Geometry: final body of the model. Coordinates: model frame, mm. A direction names the side the tool comes from. Give positions to 0.01 mm unless a question says otherwise; leave off trailing zeros. Order: outer loops, then holes, each group sorted by start corner. A loop starts at its lowest first (then second) coordinate and runs counter-clockwise, first axis right, second up. Notation, with made-up numbers: (-29.75, 37) -> (-1.75, 37) arc R19 ccw to (-1.75, 60) -> close; hole circle Ø9 at (61, 45.5). An arc over 180 degrees is marked (long way). Write item = value, one per line.
```python
from build123d import *

# Parameters (mm, degrees)
SKETCH2_R           = 7.5
SKETCH2_R_2         = 2.75
BOSS_EXTRUDE1_DEPTH = 3
SKETCH3_R           = 5.6
BOSS_EXTRUDE2_DEPTH = 4
BOSS_EXTRUDE3_DEPTH = 80
SKETCH5_W           = 29.85
SKETCH5_H           = 6.5
SKETCH5_W_2         = 3.85
BOSS_EXTRUDE4_DEPTH = 80
SKETCH6_W           = 29.85
SKETCH6_H           = 6.5
SKETCH6_W_2         = 3.85
CUT_EXTRUDE1_DEPTH  = 54.2
BOSS_EXTRUDE5_DEPTH = 22.8
SKETCH8_W           = 10.25
SKETCH8_H           = 10
SKETCH8_R           = 2.75
BOSS_EXTRUDE6_DEPTH = 5
BOSS_EXTRUDE7_DEPTH = 5
FILLET1_R           = 2.5


with BuildPart() as part:
    # Sketch2 → Boss-Extrude1 (new body)
    # profile 1 of 4: a face of its own
    with BuildSketch(Plane.XY):
        with Locations((-20, -30)):
            Circle(SKETCH2_R)
        with Locations((-20, -30)):
            Circle(SKETCH2_R_2, mode=Mode.SUBTRACT)
    # profile 2 of 4: a face of its own
    with BuildSketch(Plane.XY):
        with BuildLine():
            Line((12.5, -22.5), (-20, -22.5))
            ThreePointArc((-20, -22.5), (-14.696699141, -24.696699141), (-12.5, -30))
            ThreePointArc((-12.5, -30), (-14.696699141, -35.303300859), (-20, -37.5))
            Line((-20, -37.5), (20, -37.5))
            ThreePointArc((20, -37.5), (14.696699141, -35.303300859), (12.5, -30))
            Line((12.5, -30), (12.5, -22.5))
        make_face()
    # profile 3 of 4: a face of its own
    with BuildSketch(Plane.XY):
        with Locations((20, -30)):
            Circle(SKETCH2_R)
        with Locations((20, -30)):
            Circle(SKETCH2_R_2, mode=Mode.SUBTRACT)
    # profile 4 of 4: a face of its own
    with BuildSketch(Plane.XY):
        with BuildLine():
            Line((20, -22.5), (12.5, -22.5))
            Line((12.5, -22.5), (12.5, -30))
            ThreePointArc((12.5, -30), (14.696699141, -24.696699141), (20, -22.5))
        make_face()
    extrude(amount=BOSS_EXTRUDE1_DEPTH)

    # Sketch3 → Boss-Extrude2 (add)
    # profile 1 of 14: a face of its own
    with BuildSketch(Plane.XY.offset(3)):
        with BuildLine():
            Line((-14.4, -26.766838493), (-17.199999967, -25.150257758))
            ThreePointArc((-17.199999967, -25.150257758), (-15.150257729, -27.200000016), (-14.4, -30))
            Line((-14.4, -30), (-14.4, -26.766838493))
        make_face()
    # profile 2 of 14: a face of its own
    with BuildSketch(Plane.XY.offset(3)):
        with Locations((-20, -30)):
            Circle(SKETCH3_R)
        Polygon((-15.9, -27.632863896), (-20, -25.265727793), (-24.1, -27.632863896), (-24.1, -32.367136104), (-20, -34.734272207), (-15.9, -32.367136104), align=None, mode=Mode.SUBTRACT)
    # profile 3 of 14: a face of its own
    with BuildSketch(Plane.XY.offset(3)):
        with BuildLine():
            Line((-17.199999967, -25.150257758), (-20, -23.533676985))
            Line((-20, -23.533676985), (-22.800000033, -25.150257758))
            ThreePointArc((-22.800000033, -25.150257758), (-20, -24.4), (-17.199999967, -25.150257758))
        make_face()
    # profile 4 of 14: a face of its own
    with BuildSketch(Plane.XY.offset(3)):
        with BuildLine():
            ThreePointArc((-25.6, -30), (-24.849742271, -27.200000016), (-22.800000033, -25.150257758))
            Line((-22.800000033, -25.150257758), (-25.6, -26.766838493))
            Line((-25.6, -26.766838493), (-25.6, -30))
        make_face()
    # profile 5 of 14: a face of its own
    with BuildSketch(Plane.XY.offset(3)):
        with BuildLine():
            ThreePointArc((-22.800000033, -34.849742242), (-24.849742271, -32.799999984), (-25.6, -30))
            Line((-25.6, -30), (-25.6, -33.233161507))
            Line((-25.6, -33.233161507), (-22.800000033, -34.849742242))
        make_face()
    # profile 6 of 14: a face of its own
    with BuildSketch(Plane.XY.offset(3)):
        with BuildLine():
            ThreePointArc((-17.199999967, -34.849742242), (-20, -35.6), (-22.800000033, -34.849742242))
            Line((-22.800000033, -34.849742242), (-20, -36.466323015))
            Line((-20, -36.466323015), (-17.199999967, -34.849742242))
        make_face()
    # profile 7 of 14: a face of its own
    with BuildSketch(Plane.XY.offset(3)):
        with BuildLine():
            Line((-14.4, -33.233161507), (-14.4, -30))
            ThreePointArc((-14.4, -30), (-15.150257729, -32.799999984), (-17.199999967, -34.849742242))
            Line((-17.199999967, -34.849742242), (-14.4, -33.233161507))
        make_face()
    # profile 8 of 14: a face of its own
    with BuildSketch(Plane.XY.offset(3)):
        with BuildLine():
            Line((25.6, -26.766838493), (22.800000033, -25.150257758))
            ThreePointArc((22.800000033, -25.150257758), (24.849742271, -27.200000016), (25.6, -30))
            Line((25.6, -30), (25.6, -26.766838493))
        make_face()
    # profile 9 of 14: a face of its own
    with BuildSketch(Plane.XY.offset(3)):
        with Locations((20, -30)):
            Circle(SKETCH3_R)
        Polygon((24.1, -27.632863896), (20, -25.265727793), (15.9, -27.632863896), (15.9, -32.367136104), (20, -34.734272207), (24.1, -32.367136104), align=None, mode=Mode.SUBTRACT)
    # profile 10 of 14: a face of its own
    with BuildSketch(Plane.XY.offset(3)):
        with BuildLine():
            Line((22.800000033, -25.150257758), (20, -23.533676985))
            Line((20, -23.533676985), (17.199999967, -25.150257758))
            ThreePointArc((17.199999967, -25.150257758), (20, -24.4), (22.800000033, -25.150257758))
        make_face()
    # profile 11 of 14: a face of its own
    with BuildSketch(Plane.XY.offset(3)):
        with BuildLine():
            ThreePointArc((14.4, -30), (15.150257729, -27.200000016), (17.199999967, -25.150257758))
            Line((17.199999967, -25.150257758), (14.4, -26.766838493))
            Line((14.4, -26.766838493), (14.4, -30))
        make_face()
    # profile 12 of 14: a face of its own
    with BuildSketch(Plane.XY.offset(3)):
        with BuildLine():
            ThreePointArc((17.199999967, -34.849742242), (15.150257729, -32.799999984), (14.4, -30))
            Line((14.4, -30), (14.4, -33.233161507))
            Line((14.4, -33.233161507), (17.199999967, -34.849742242))
        make_face()
    # profile 13 of 14: a face of its own
    with BuildSketch(Plane.XY.offset(3)):
        with BuildLine():
            ThreePointArc((22.799999796, -34.849742379), (19.999999863, -35.6), (17.199999967, -34.849742242))
            Line((17.199999967, -34.849742242), (20, -36.466323015))
            Line((20, -36.466323015), (22.799999796, -34.849742379))
        make_face()
    # profile 14 of 14: a face of its own
    with BuildSketch(Plane.XY.offset(3)):
        with BuildLine():
            Line((25.6, -33.233161507), (25.6, -30))
            ThreePointArc((25.6, -30), (24.849742202, -32.800000102), (22.799999796, -34.849742379))
            Line((22.799999796, -34.849742379), (25.6, -33.233161507))
        make_face()
    extrude(amount=BOSS_EXTRUDE2_DEPTH)

    # Sketch4 → Boss-Extrude3 (add)
    with BuildSketch(Plane.XY.offset(3)):
        Polygon((-14.4, -26.766838493), (-14.4, -22.5), (-11.4, -22.5), (-11.4, -37.5), (-14.4, -37.5), align=None)
        Polygon((14.4, -30), (14.4, -22.5), (11.4, -22.5), (11.4, -37.5), (14.4, -37.5), align=None)
    extrude(amount=BOSS_EXTRUDE3_DEPTH)

    # Sketch5 → Boss-Extrude4 (add)
    with BuildSketch(Plane.ZY.offset(-11.4)):
        with Locations((63.075, -34.25)):
            Rectangle(SKETCH5_W, SKETCH5_H)
        with Locations((42.925, -34.25)):
            Rectangle(SKETCH5_W_2, SKETCH5_H)
    extrude(amount=BOSS_EXTRUDE4_DEPTH)

    # Sketch6 → Cut-Extrude1 (cut)
    with BuildSketch(Plane.ZY.offset(68.6)):
        with Locations((63.075, -34.25)):
            Rectangle(SKETCH6_W, SKETCH6_H)
        with Locations((42.925, -34.25)):
            Rectangle(SKETCH6_W_2, SKETCH6_H)
    extrude(amount=-CUT_EXTRUDE1_DEPTH, mode=Mode.SUBTRACT)

    # Sketch7 → Boss-Extrude5 (add)
    with BuildSketch(Plane.ZY.offset(-11.4)):
        Polygon((78, -31), (78, -22.5), (83, -22.5), (83, -37.5), (78, -37.5), align=None)
    extrude(amount=BOSS_EXTRUDE5_DEPTH)

    # Sketch8 → Boss-Extrude6 (add)
    # profile 1 of 2: a face of its own
    with BuildSketch(Plane.XZ.offset(22.5)):
        with Locations((-19.525, 59.5)):
            Rectangle(SKETCH8_W, SKETCH8_H)
        with Locations((-19.525, 59.5)):
            Circle(SKETCH8_R, mode=Mode.SUBTRACT)
    # profile 2 of 2: a face of its own
    with BuildSketch(Plane.XZ.offset(22.5)):
        with Locations((19.525, 59.5)):
            Rectangle(SKETCH8_W, SKETCH8_H)
        with Locations((19.525, 59.5)):
            Circle(SKETCH8_R, mode=Mode.SUBTRACT)
    extrude(amount=BOSS_EXTRUDE6_DEPTH)

    # Sketch10 → Boss-Extrude7 (add)
    with BuildSketch(Plane(origin=(0, -22.5, 0), x_dir=(1, 0, 0), z_dir=(0, 1, 0))):
        Polygon((-10, -38.8), (10, -38.8), (11.4, -38.8), (11.4, -35.8), (-11.4, -35.8), (-11.4, -38.8), align=None)
    extrude(amount=-BOSS_EXTRUDE7_DEPTH)

    # Fillet1
    fillet1_edges = [part.edges().sort_by_distance(p)[0] for p in [
        (-14.4, -30, 83),
        (14.4, -30, 83),
    ]]
    fillet(fillet1_edges, radius=FILLET1_R)


solid = part.part
```
1) Section query D-D (z = 11.5). Output: boundary loops of the cut face in (x, y), plus the area to 3 significant figures.
Check sheet entries:
outline = (-14.4, -37.5) -> (-11.4, -37.5) -> (-11.4, -22.5) -> (-14.4, -22.5) -> close; (11.4, -37.5) -> (14.4, -37.5) -> (14.4, -22.5) -> (11.4, -22.5) -> close
area = 90.0 mm²
2) Section query A-A (y = -28.75). Count the separate pieces of the cut face and the enclosed holes in it, plus the area to 3 significant figures.
Check sheet entries:
separate_pieces = 3
enclosed_holes = 1
area = 750 mm²
3) First-contact query: P1, Ø1, axis at y = -32.5, z = 70, coming from the -X side; P2, Ø5, axis at x = 13, y = -28, coming from the -Z side; P3, Ø1, axis at y = -32, z = 12, coming from the +X side; P4, Ø3, axis at x = -0.5, z = 42.5, coming from the +Y side. Flat tips, straight axial feed; report the tip coordinate or a pass-through.
Check sheet entries:
P1 = -14.4
P2 = 0
P3 = 14.4
P4 = -31
4) Reachability of faces 4 (the face through (26, -29, 3)), 5 (the face through (0, -34, 48.15)), 6 (the face through (19, -25, 54.5)) from +Z, -Z, +X, -X, +Y, -Y: full face, straight path, thin tool, end or side. Return the list, or none.
Check sheet entries:
face_4 = none
face_5 = +Y, -Y
face_6 = +X, +Y, -Y
5) Mould query, pull axis X, two halves, no side actions, for faces 1 (the face through (-18, -26, 7)), 2 (the face through (22.02, -33.57, 4.97)), 3 (the face through (-13.687, -30.105, 82.248)). Classes: +X half, -X half, draft (parallel to the pull), parting line (faces both ways), or undercut.
Check sheet entries:
face_1 = draft
face_2 = undercut
face_3 = -X half
6) Section query B-B (x = -5.5). Output: boundary loops of the cut face in (y, z).
Check sheet entries:
outline = (-37.5, 0) -> (-22.5, 0) -> (-22.5, 3) -> (-37.5, 3) -> close; (-37.5, 41) -> (-31, 41) -> (-31, 44.85) -> (-37.5, 44.85) -> close; (-37.5, 48.15) -> (-31, 48.15) -> (-31, 78) -> (-22.5, 78) -> (-22.5, 83) -> (-37.5, 83) -> close; (-27.5, 35.8) -> (-22.5, 35.8) -> (-22.5, 38.8) -> (-27.5, 38.8) -> close
7) Section query C-C (z = 59.5). Output: boundary loops of the cut face in (x, y) (3 decimals), plus the area to 3 significant figures.
Check sheet entries:
outline = (-24.65, -27.5) -> (-22.275, -27.5) -> (-22.275, -22.5) -> (-24.65, -22.5) -> close; (-16.775, -27.5) -> (-14.4, -27.5) -> (-14.4, -37.5) -> (14.4, -37.5) -> (14.4, -27.5) -> (16.775, -27.5) -> (16.775, -22.5) -> (11.4, -22.5) -> (11.4, -31) -> (-11.4, -31) -> (-11.4, -22.5) -> (-16.775, -22.5) -> close; (22.275, -27.5) -> (24.65, -27.5) -> (24.65, -22.5) -> (22.275, -22.5) -> close
area = 286 mm²
8) Line query: line 1 (Z direction, x = -3.5, y = -36.25); line 2 (Z direction, x = -0.5, y = -24.5); line 3 (X direction, y = -30.5, z = 69). Output: solid intervals per line, ascending. Write a range as from..to.
Check sheet entries:
line_1 = 0..3, 41..44.85, 48.15..83
line_2 = 0..3, 35.8..38.8, 78..83
line_3 = -14.4..-11.4, 11.4..14.4
